Check sheet for the modelled part. Datum: model origin and axes. Units: mm. Face numbers are marked on the shaded views. A direction names the side the tool comes from. Coordinates: 2 decimals unless noted, no trailing zeros. Loops run counter-clockwise (first coordinate to the right, second up) from the corner with the lowest first, then second, coordinate; pieces in that order, holes last. Notation, with made-up numbers: M -22.75,-20.75 L 2.25,-20.75 A12 cw 2.25,-14.75 Z; hole C 1,-24 d5. An arc over 180 degrees is marked long. Use CSV: the item, a comma, the result in double quotes. Start each with the question number.
(1) Section check B-B on x = 42.5. Record the cut outline in (y, z), and give its area (3 significant figures).
(2) Section check A-A on x = 63.5. Record the cut outline in (y, z).
(3) Set-up check for the marked faces 1, 2 and 3: record each of +Z, -Z, +X, -X, +Y, -Y from which the full face is reachable in a straight line by a thin tool's end or side.
(4) Go/stop test with flat-tipped pins: pin 1 Ø2 at (x, z) = (114.5, -19) entering from -Y; pin 2 Ø6 at (x, y) = (96, 49) entering from -Z; pin 3 Ø0.9 at (x, y) = (68.5, -16) entering from -Z. Record where each tip stops, or that it passes through.
(5) Scan lines: line 1 (Y direction, x = 138, z = 0); line 2 (Y direction, x = 79.5, z = 0); line 3 (Y direction, x = 92.5, z = -21). Record each from-to range of solid material in increasing order.
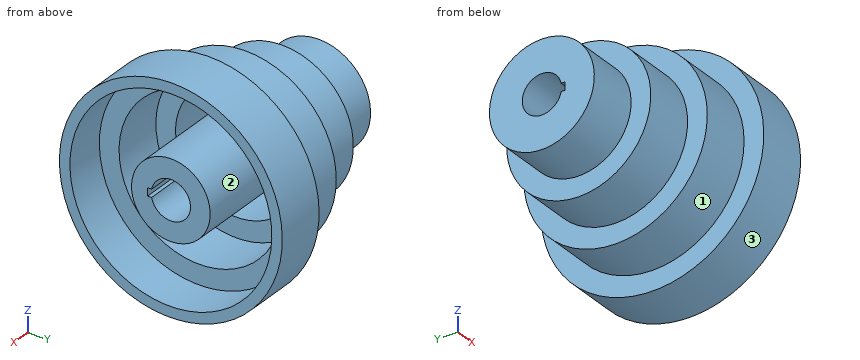
from build123d import *

# Parameters (mm, degrees)
CUT_EXTRUDE1_REACH = 202.125


with BuildPart() as part:
    # Sketch1 → Revolve1 (revolve)
    with BuildSketch(Plane(origin=(0, 0, 0), x_dir=(1, 0, 0), z_dir=(0, 1, 0)), mode=Mode.PRIVATE) as revolve1_sk:
        Polygon((0, 15), (0, 40), (40, 40), (40, 55), (80, 55), (80, 70), (120, 70), (120, 85), (160, 85), (160, 77), (128, 77), (128, 62), (88, 62), (88, 47), (48, 47), (48, 30), (160, 30), (160, 15), align=None)
    revolve(revolve1_sk.sketch.rotate(Axis((-116.687976722, 0, 0), (1, 0, 0)), 180), axis=Axis((-116.687976722, 0, 0), (1, 0, 0)))

    # Sketch2 → Cut-Extrude1 (cut, up to next)
    with BuildSketch(Plane.ZY, mode=Mode.PRIVATE) as cut_extrude1_sk1:
        with BuildLine():
            Line((-3, -14.696938457), (-3, -17.696938457))
            Line((-3, -17.696938457), (3, -17.696938457))
            Line((3, -17.696938457), (3, -14.696938457))
            ThreePointArc((3, -14.696938457), (0, -15), (-3, -14.696938457))
        make_face()
    cut_extrude1_tool1 = extrude(cut_extrude1_sk1.sketch, amount=-CUT_EXTRUDE1_REACH, mode=Mode.PRIVATE) & part.part
    add(cut_extrude1_tool1.solids().sort_by_distance((0, -16.29671, 0))[0], mode=Mode.SUBTRACT)


solid = part.part
Outcome:
1,outline,"C 0,0 d110; hole M -17.7,-3 L -14.7,-3 A15 ccw long -14.7,3 L -17.7,3 Z"
1,area,"8,780 mm²"
2,outline,"C 0,0 d110; C 0,0 d60; hole C 0,0 d94; hole M -17.7,-3 L -14.7,-3 A15 ccw long -14.7,3 L -17.7,3 Z"
3,face 1,"-X"
3,face 2,"+X"
3,face 3,"+X, -X"
4,pin 1,"stops at y = -67.65"
4,pin 2,"stops at z = -52.76"
4,pin 3,"stops at z = -52.76"
5,line 1,"y = -85 to -77, -30 to -17.7, 15 to 30, 77 to 85"
5,line 2,"y = -55 to -47, -30 to -17.7, 15 to 30, 47 to 55"
5,line 3,"y = -66.78 to -58.34, -21.42 to 21.42, 58.34 to 66.78"
